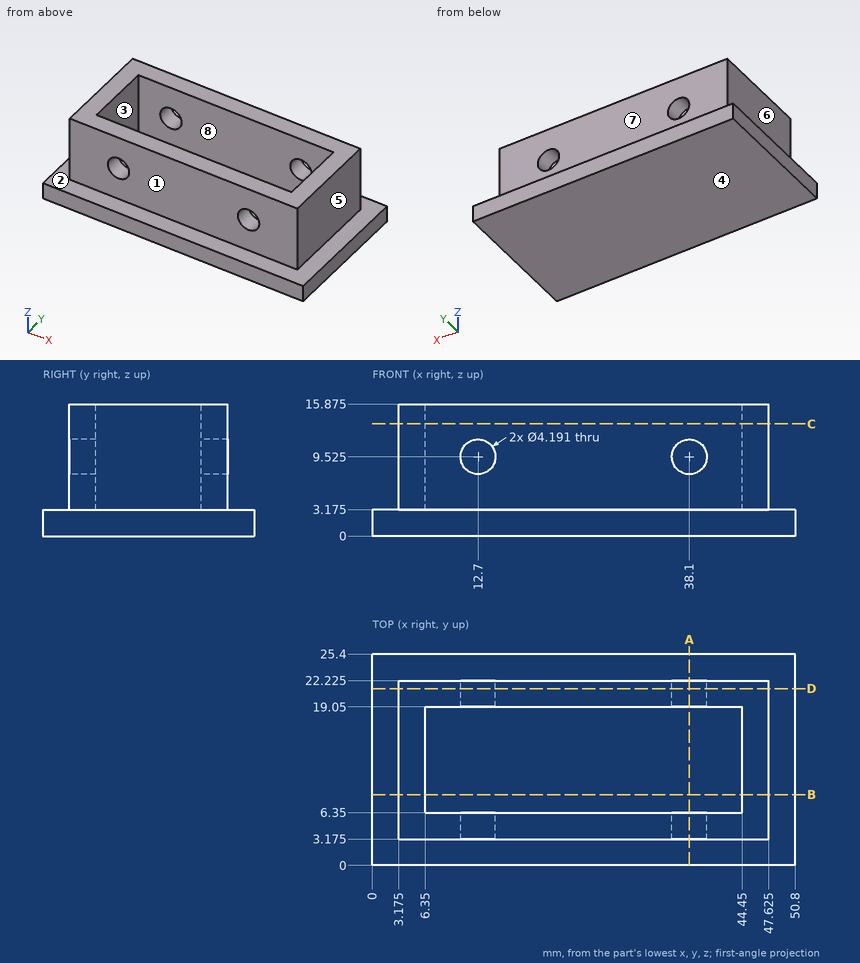
Part print with two shaded views. Sizes in mm from the minimum x, y, z corner. A direction names the side the tool comes from. Round coordinates to 2 decimals unless told otherwise and drop trailing zeros. Loops run counter-clockwise (first coordinate to the right, second up) from the corner with the lowest first, then second, coordinate; pieces in that order, holes last.
1. Two-plate mould, pull along Y, no slides. Class the marked faces 1, 2 and 3: pulls with the +Y half, pulls with the -Y half, needs draft (parallel to the pull), parting line crosses it, or undercut.
Solutions:
face 1: pulls with the -Y half
face 2: needs draft
face 3: undercut
2. Flat gauge pins, fed straight in: pin 1 (5.5 mm diameter, centred on x = 38.1, z = 9.525, fed in from -Y) (3 decimals); pin 2 (4 mm diameter, centred on x = 35, y = 10.5, fed in from +Z) (3 decimals); pin 3 (1 mm diameter, centred on y = 6.5, z = 6, fed in from +X) (3 decimals). Where does each tip first touch, or does it go through?
Solutions:
pin 1: stops at y = 3.175
pin 2: stops at z = 3.175
pin 3: stops at x = 47.625
3. Drill centre lines: line 1 along X through (y, z) = (19, 6) (3 decimals); line 2 along Y through (x, z) = (29.5, 10) (3 decimals); line 3 along Z through (x, y) = (38.1, 4) (1 decimal). Where is each one in solid material? Low to high.
Solutions:
line 1: x = 3.175 to 6.35, 44.45 to 47.625
line 2: y = 3.175 to 6.35, 19.05 to 22.225
line 3: z = 0 to 7.4, 11.6 to 15.9
4. Slice it at D-D (y = 21.25). Give the cut face in (x, z) (1 decimal).
Solutions:
outline: (0, 0) - (50.8, 0) - (50.8, 3.2) - (47.6, 3.2) - (47.6, 15.9) - (3.2, 15.9) - (3.2, 3.2) - (0, 3.2) - close; hole circle Ø4.2 at (12.7, 9.5); hole circle Ø4.2 at (38.1, 9.5)
5. Slice it at A-A (x = 38.1). Count the separate pieces of the cut face and the enclosed holes in it, and give its area (3 significant figures).
Solutions:
separate pieces: 3
enclosed holes: 0
area: 135 mm2
6. Slice it at B-B (y = 8.5). Give the cut face in (x, z) (3 decimals).
Solutions:
outline: (0, 0) - (50.8, 0) - (50.8, 3.175) - (47.625, 3.175) - (47.625, 15.875) - (44.45, 15.875) - (44.45, 3.175) - (6.35, 3.175) - (6.35, 15.875) - (3.175, 15.875) - (3.175, 3.175) - (0, 3.175) - close
7. 3-axis set-ups, long thin cutter, end or side, ignore diameter. For the marked faces 4, 5, 6, 7 and 8: which of +Z, -Z, +X, -X, +Y, -Y reach the whole face in a straight line?
Solutions:
face 4: -Z, +X, -X, +Y, -Y
face 5: +Z, +X, +Y, -Y
face 6: +Z, -X, +Y, -Y
face 7: +Z, +X, -X, +Y
face 8: +Z
8. Slice it at C-C (z = 13.5). Give the cut face in (x, y) (3 decimals), and give its area (3 significant figures).
Solutions:
outline: (3.175, 3.175) - (47.625, 3.175) - (47.625, 22.225) - (3.175, 22.225) - close; hole (6.35, 6.35) - (44.45, 6.35) - (44.45, 19.05) - (6.35, 19.05) - close
area: 363 mm2
